```python
from build123d import *

# Parameters (mm, degrees)
SKETCH1_R             = 6
SKETCH1_R_2           = 2.5
BOSS_EXTRUDE1_DEPTH   = 20
BOSS_EXTRUDE2_DEPTH   = 4
SKETCH3_W             = 2.5
SKETCH3_H             = 6
CUT_EXTRUDE1_DEPTH    = 15
BODY_MOVE_COPY1_ANGLE = 180
BOSS_EXTRUDE3_START   = 1
SKETCH4_R             = 6
BOSS_EXTRUDE3_DEPTH   = 1
SKETCH5_R             = 4.5
BOSS_EXTRUDE4_DEPTH   = 5
SKETCH6_R             = 3.5
CUT_EXTRUDE2_DEPTH    = 5
SKETCH7_W             = 1.05927087
SKETCH7_H             = 5
SKETCH7_W_2           = 1.30456568
BOSS_EXTRUDE5_DEPTH   = 21
SKETCH8_R             = 1.75
CUT_EXTRUDE3_DEPTH    = 39
SKETCH9_R             = 1.5
CUT_EXTRUDE4_DEPTH    = 37.827299731
SKETCH11_R            = 1.5
CUT_EXTRUDE5_DEPTH    = 37.827299731


with BuildPart() as part:
    # Sketch1 → Boss-Extrude1 (new body)
    with BuildSketch(Plane.XY):
        Circle(SKETCH1_R)
        Circle(SKETCH1_R_2, mode=Mode.SUBTRACT)
    extrude(amount=BOSS_EXTRUDE1_DEPTH)

    # Sketch2 → Boss-Extrude2 (add, symmetric)
    with BuildSketch(Plane(origin=(0, 0, 0), x_dir=(0, 0, -1), z_dir=(1, 0, 0))):
        Polygon((-20, 6), (-20, 3), (0, 3), (0, 30), (-6, 30), align=None)
    extrude(amount=BOSS_EXTRUDE2_DEPTH, both=True)

    # Sketch3 → Cut-Extrude1 (cut)
    with BuildSketch(Plane(origin=(0, 30, 0), x_dir=(1, 0, 0), z_dir=(0, 1, 0))):
        with Locations((-2.75, -3)):
            Rectangle(SKETCH3_W, SKETCH3_H)
        with Locations((2.75, -3)):
            Rectangle(SKETCH3_W, SKETCH3_H)
    extrude(amount=-CUT_EXTRUDE1_DEPTH, mode=Mode.SUBTRACT)


with BuildPart() as body_2:
    # Body-Move/Copy1: copy of part
    add(part.part.rotate(Axis((0, 0, 0), (0, 0, 1)), BODY_MOVE_COPY1_ANGLE))


with BuildPart() as part_1:
    add(part.part)

    add(body_2.part)  # Boss-Extrude3 merges body 2
    # Sketch4 → Boss-Extrude3 (add)
    with BuildSketch(Plane(origin=(0, 0, 0), x_dir=(-1, 0, 0), z_dir=(0, 0, -1)).offset(BOSS_EXTRUDE3_START)):
        Circle(SKETCH4_R)
    extrude(amount=-BOSS_EXTRUDE3_DEPTH)

    # Sketch5 → Boss-Extrude4 (add)
    with BuildSketch(Plane(origin=(0, 0, -1), x_dir=(-1, 0, 0), z_dir=(0, 0, -1))):
        Circle(SKETCH5_R)
    extrude(amount=BOSS_EXTRUDE4_DEPTH)

    # Sketch6 → Cut-Extrude2 (cut)
    with BuildSketch(Plane(origin=(0, 0, -6), x_dir=(-1, 0, 0), z_dir=(0, 0, -1))):
        Circle(SKETCH6_R)
    extrude(amount=-CUT_EXTRUDE2_DEPTH, mode=Mode.SUBTRACT)

    # Sketch7 → Boss-Extrude5 (add)
    with BuildSketch(Plane.XY.offset(20)):
        with Locations((-5.470364565, 0)):
            Rectangle(SKETCH7_W, SKETCH7_H)
        with Locations((5.34771716, 0)):
            Rectangle(SKETCH7_W_2, SKETCH7_H)
    extrude(amount=-BOSS_EXTRUDE5_DEPTH)

    # Sketch8 → Cut-Extrude3 (cut, through all)
    with BuildSketch(Plane.ZY.offset(6)):
        with Locations((5, 0)):
            Circle(SKETCH8_R)
        with Locations((15, 0)):
            Circle(SKETCH8_R)
    extrude(amount=-CUT_EXTRUDE3_DEPTH, mode=Mode.SUBTRACT)

    # Sketch9 → Cut-Extrude4 (cut, through all)
    with BuildSketch(Plane.ZY.offset(1.5)):
        with Locations((3, 17.5)):
            Circle(SKETCH9_R)
        with Locations((3, 22.5)):
            Circle(SKETCH9_R)
        with Locations((3, 27.5)):
            Circle(SKETCH9_R)
    extrude(amount=-CUT_EXTRUDE4_DEPTH, mode=Mode.SUBTRACT)

    # Sketch11 → Cut-Extrude5 (cut, through all)
    with BuildSketch(Plane.ZY.offset(1.5)):
        with Locations(Location((3, -17.5, 0), (0, 0, 270))):
            Circle(SKETCH11_R)
        with Locations(Location((3, -22.5, 0), (0, 0, 270))):
            Circle(SKETCH11_R)
        with Locations(Location((3, -27.5, 0), (0, 0, 270))):
            Circle(SKETCH11_R)
    extrude(amount=-CUT_EXTRUDE5_DEPTH, mode=Mode.SUBTRACT)


solid = part_1.part
```
Check sheet for the modelled part. Datum: model origin and axes. Units: mm. A direction names the side the tool comes from. Round coordinates to 2 decimals unless told otherwise and drop trailing zeros. Order: outer loops, then holes, each group sorted by start corner. A loop starts at its lowest first (then second) coordinate and runs counter-clockwise, first axis right, second up. Notation, with made-up numbers: (-20.5, -32.75) - (28.5, -32.75) arc R30 cw to (28.5, -4.75) - close; hole circle Ø7 at (13, 66). An arc over 180 degrees is marked (long way). Write item = value, one per line.
Q1. Section check B-B (y = -22.5). Record the boundary of the cut face in (x, z) (3 decimals), and give its area (3 significant figures).
Computed:
outline = (-4, 6) - (-1.5, 6) - (-1.5, 4.5) - (1.5, 4.5) - (1.5, 6) - (4, 6) - (4, 10.375) - (-4, 10.375) - close; (-1.5, 0) - (1.5, 0) - (1.5, 1.5) - (-1.5, 1.5) - close
area = 44.0 mm^2
Q2. Section check D-D (z = 18.25). Record the boundary of the cut face in (x, y).
Computed:
outline = (-6, -2.5) - (-5.45, -2.5) arc R6 ccw to (-4, -4.47) - (-4, -9) - (4, -9) - (4, -4.47) arc R6 ccw to (5.45, -2.5) - (6, -2.5) - (6, 2.5) - (5.45, 2.5) arc R6 ccw to (4, 4.47) - (4, 9) - (-4, 9) - (-4, 4.47) arc R6 ccw to (-5.45, 2.5) - (-6, 2.5) - close; hole circle Ø5 at (0, 0)
Q3. Tool access check on faces 1 (the face through (0, 30, 3)), 2 (the face through (3, 15, 3)), 3 (the face through (1.5, -24.3, 3)), 4 (the face through (4, 12, 8)), 5 (the face through (-3, 23, 6)). Record the directions out of +Z, -Z, +X, -X, +Y, -Y that give a thin tool (end or side, any length) a straight path to the whole face; none if there is none.
Computed:
face_1 = +Z, -Z, +X, -X, +Y
face_2 = -Z, +X, +Y
face_3 = -Z, +X, -Y
face_4 = +Z, -Z, +X, +Y
face_5 = -Z, -X, +Y
Q4. Go/stop test with flat-tipped pins: pin 1 (1.5 mm diameter, centred on x = 4, y = 14, fed in from +Z); pin 2 (12 mm diameter, centred on y = -17, z = 3.5, fed in from -X); pin 3 (1 mm diameter, centred on y = -10, z = 11, fed in from +X); pin 4 (1.5 mm diameter, centred on x = -5, y = -9, fed in from +Z). Record where each tip stops, or that it passes through.
Computed:
pin_1 = 15.77
pin_2 = -4
pin_3 = 4
pin_4 = through
Q5. Thickness scan on line 1 along Z through (x, y) = (-4.8, 0); line 2 along X through (y, z) = (-2, 9.75); line 3 along X through (y, z) = (0, 1.5). Record the ranges inside material, lowest first.
Computed:
line_1 = -1 to 3.25, 6.75 to 13.25, 16.75 to 20
line_2 = -6 to -1.5, 1.5 to 6
line_3 = -6 to -2.5, 2.5 to 6
Q6. Section check A-A (x = 0). Record the boundary of the cut face in (y, z), and give its area (3 significant figures).
Computed:
outline = (-30, 0) - (-6, 0) - (-6, -1) - (-4.5, -1) - (-4.5, -6) - (-3.5, -6) - (-3.5, -1) - (3.5, -1) - (3.5, -6) - (4.5, -6) - (4.5, -1) - (6, -1) - (6, 0) - (30, 0) - (30, 6) - (6, 20) - (2.5, 20) - (2.5, 0) - (-2.5, 0) - (-2.5, 20) - (-6, 20) - (-30, 6) - close; hole circle Ø3 at (-27.5, 3); hole circle Ø3 at (-22.5, 3); hole circle Ø3 at (-17.5, 3); hole circle Ø3 at (17.5, 3); hole circle Ø3 at (22.5, 3); hole circle Ø3 at (27.5, 3)
area = 744 mm^2
Q7. Draft check along Y on faces 6 (the face through (0, 0, 0)), 7 (the face through (0, -26, 3)), 8 (the face through (-3, -15, 3)), 9 (the face through (-1.5, -24.3, 3)). Enter one of: pulls with the +Y half, pulls with the -Y half, needs draft (parallel to the pull), parting line crosses it, or undercut.
Computed:
face_6 = undercut
face_7 = undercut
face_8 = pulls with the -Y half
face_9 = needs draft
Q8. Section check C-C (z = 15). Record the boundary of the cut face in (x, y), and give its area (3 significant figures).
Computed:
outline = (-6, -2.5) - (-5.45, -2.5) arc R6 ccw to (-4, -4.47) - (-4, -14.57) - (4, -14.57) - (4, -4.47) arc R6 ccw to (5.45, -2.5) - (6, -2.5) - (6, -1.75) - (1.79, -1.75) arc R2.5 cw to (-1.79, -1.75) - (-6, -1.75) - close; (-6, 1.75) - (-1.79, 1.75) arc R2.5 cw to (1.79, 1.75) - (6, 1.75) - (6, 2.5) - (5.45, 2.5) arc R6 ccw to (4, 4.47) - (4, 14.57) - (-4, 14.57) - (-4, 4.47) arc R6 ccw to (-5.45, 2.5) - (-6, 2.5) - close
area = 214 mm^2
